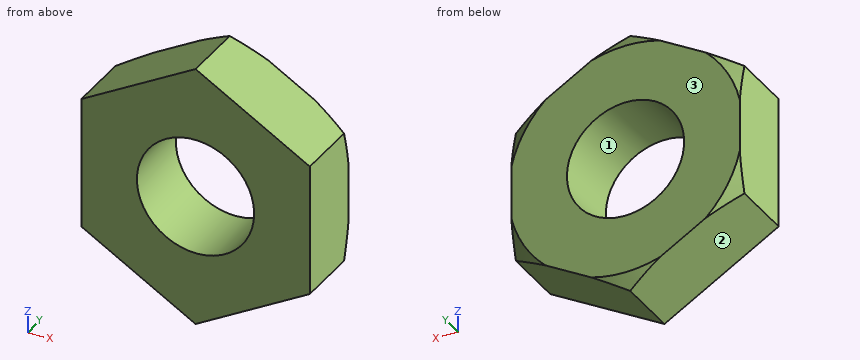
Autodesk Inventor part; units mm, degrees
ref_plane "YZ Plane" through (0, 0, 0) normal (1, 0, 0) x (0, 1, 0)
ref_plane "XZ Plane" through (0, 0, 0) normal (0, 1, 0) x (-1, 0, 0)
ref_plane "XY Plane" through (0, 0, 0) normal (0, 0, 1) x (1, 0, 0)
sketch "スケッチ1" plane through (0, 0, 0) normal (0, 0, 1) x (1, 0, 0)
  line L0 (2, 1.2) -> (4, 1.2)
  line L1 (4.5, 0.9113) -> (4.5, -1.2)
  line L2 (4.5, -1.2) -> (2, -1.2)
  line L3 (2, -1.2) -> (2, 1.2)
  line L4 (0, 1.2) -> (0, -1.2)
  line L5 (4, 1.2) -> (4.5, 0.9113)
  point P0 (0, 0)
  dimension "d0" = 1.2
  dimension "d1" = 2.4
  dimension "d2" = 2
  dimension "d3" = 4.5
  dimension "d4" = 2
  dimension "d5" = 30
revolve "回転1" add sketch "スケッチ1" angle 360 about axis through (0, 1.2, 0) along (0, -1, 0)
sketch "スケッチ2" plane through (0, 1.2, 0) normal (0, 1, 0) x (1, 0, 0)
  circle A0 centre (0, 0) radius 2
  line L0 (0, 4.5) -> (3.8971, 2.25)
  line L1 (3.8971, 2.25) -> (3.8971, -2.25)
  line L2 (3.8971, -2.25) -> (0, -4.5)
  line L3 (0, -4.5) -> (-3.8971, -2.25)
  line L4 (-3.8971, -2.25) -> (-3.8971, 2.25)
  line L5 (-3.8971, 2.25) -> (0, 4.5)
  dimension "d7" = 4.5
extrude "押し出し1" cut sketch "スケッチ2" against normal blind 2.4 keep common part
thread "ねじ2"
properties material "ステンレス鋼"
Work out the finished part from the listing and answer in its coordinate system (mm). Face numbers are marked on the shaded views. Coordinates: 2 decimals unless noted, no trailing zeros. Loops run counter-clockwise (first coordinate to the right, second up) from the corner with the lowest first, then second, coordinate; pieces in that order, holes last. Notation, with made-up numbers: M -6.5,80 L 2.5,80 A20 ccw 2.5,105 Z; hole C 19,50.25 d11. An arc over 180 degrees is marked long. Answer in a Markdown table with one row per item. Add a question column.
1. Consider L1, parallel to X at y = -0.4, z = 1; L2, parallel to X at y = 0.1, z = 1.25; L3, parallel to Z at x = 0.5, y = -0.65. Determine where each line is inside the solid, lowest interval first.
2. Find section A-A, the plane z = 0. Write down the section's boundary in (x, y), then the cut area to 3 significant figures.
3. The mould has two halves that part along Z. Classify the marked faces 1, 2 and 3: pulls with the +Z half, pulls with the -Z half, needs draft (parallel to the pull), parting line crosses it, or undercut.
4. Find section B-B, the plane y = 0. Write down the section's boundary in (x, z).
5. Find section C-C, the plane x = 1.5. Write down the section's boundary in (y, z), then the cut area to 3 significant figures.
Reported:
| question | item | result |
|---|---|---|
| 1 | L1 | x = -3.9 to -1.73, 1.73 to 3.9 |
| 1 | L2 | x = -3.9 to -1.56, 1.56 to 3.9 |
| 1 | L3 | z = -4.21 to -1.94, 1.94 to 4.21 |
| 2 | outline | M -3.9,-1.2 L -2,-1.2 L -2,1.2 L -3.9,1.2 Z; M 2,-1.2 L 3.9,-1.2 L 3.9,1.2 L 2,1.2 Z |
| 2 | area | 9.11 mm^2 |
| 3 | face 1 | undercut |
| 3 | face 2 | pulls with the -Z half |
| 3 | face 3 | needs draft |
| 4 | outline | M -3.9,-2.25 L 0,-4.5 L 3.9,-2.25 L 3.9,2.25 L 0,4.5 L -3.9,2.25 Z; hole C 0,0 d4 |
| 5 | outline | M -1.2,-3.63 L 1.2,-3.63 L 1.2,-1.32 L -1.2,-1.32 Z; M -1.2,1.32 L 1.2,1.32 L 1.2,3.63 L -1.2,3.63 Z |
| 5 | area | 11.1 mm^2 |
